```python
from build123d import *

# Parameters (mm, degrees)
SZKIC1_W                    = 28
SZKIC1_H                    = 16
DODANIE_WYCI_GNI_CIE1_DEPTH = 10.4
SZKIC2_R                    = 1.5
WYTNIJ_WYCI_GNI_CIE1_DEPTH  = 10.4
ZAOKR_GLENIE1_R             = 2.5
DODANIE_WYCI_GNI_CIE2_START = -2.5
DODANIE_WYCI_GNI_CIE2_DEPTH = 5
SZKIC5_R                    = 2.229172114
DODANIE_WYCI_GNI_CIE3_DEPTH = 5


with BuildPart() as part:
    # Szkic1 → Dodanie-wyciągnięcie1 (new body)
    with BuildSketch(Plane.XY):
        with Locations((14, 8)):
            Rectangle(SZKIC1_W, SZKIC1_H)
    extrude(amount=DODANIE_WYCI_GNI_CIE1_DEPTH)

    # Szkic2 → Wytnij-wyciągnięcie1 (cut)
    with BuildSketch(Plane.XY.offset(10.4)):
        with Locations((3, 3)):
            Circle(SZKIC2_R)
        with Locations((25, 13)):
            Circle(SZKIC2_R)
    extrude(amount=-WYTNIJ_WYCI_GNI_CIE1_DEPTH, mode=Mode.SUBTRACT)

    # Zaokrąglenie1
    zaokr_glenie1_edges = [part.edges().sort_by_distance(p)[0] for p in [
        (0, 16, 5.2),
        (28, 16, 5.2),
        (28, 0, 5.2),
        (0, 0, 5.2),
    ]]
    fillet(zaokr_glenie1_edges, radius=ZAOKR_GLENIE1_R)

    # Szkic4 → Dodanie-wyciągnięcie2 (add)
    with BuildSketch(Plane.XY.offset(10.4).offset(DODANIE_WYCI_GNI_CIE2_START)):
        Polygon((17.360184227, 16), (-9.374532536, 25.006750185), (-9.835766296, 23.637671029), (15.248549739, 15.186929991), align=None)
    extrude(amount=-DODANIE_WYCI_GNI_CIE2_DEPTH)

    # Szkic5 → Dodanie-wyciągnięcie3 (add)
    with BuildSketch(Plane.XY.offset(7.9)):
        with Locations((-8.559972621, 24.732330309)):
            Circle(SZKIC5_R)
    extrude(amount=-DODANIE_WYCI_GNI_CIE3_DEPTH)


solid = part.part
```
Verification items for the finished model (mm, model axes). A direction names the side the tool comes from. Round coordinates to 2 decimals unless told otherwise and drop trailing zeros. Write each loop counter-clockwise with the first axis right and the second up, starting at its lowest first coordinate (ties: lowest second). Pieces come first, ordered by that corner, then holes. Notation, with made-up numbers: (-18, -6) -> (39, -6) arc R6 ccw to (39, 3) -> close; hole circle Ø2 at (14, 78). An arc over 180 degrees is marked (long way). Write each question's results on one line, items separated by ' | '. Start each with the question number.
1. Depth check by flat-ended pin: P1, Ø3, axis at x = 8.5, z = 3, coming from the +Y side; P2, Ø3.5, axis at x = 9.5, y = 22.5, coming from the -Z side; P3, Ø3.5, axis at x = 25, y = 13, coming from the +Z side; P4, Ø5, axis at y = 6, z = 5.5, coming from the -X side. Enter the tip coordinate at first touch or a pass-through.
2. Cross-section at A-A (z = 7.25). Enter the section's corners in (x, y), then the cut area to 3 significant figures.
3. Material ranges on probe 1 along Y at (x, z) = (25, 7.5); probe 2 along Y at (x, z) = (3, 5); probe 3 along Y at (x, z) = (10, 7), recorded low to high. Write a range as from..to.
4. Draft check along Y on faces 6 (the flat face through (0, 21, 7.9)), 7 (the cylindrical face through (27.248, 0.713, 5.273)), 8 (the cylindrical face through (27.248, 15.287, 5.273)), 9 (the cylindrical face through (3.69, 1.67, 5.27)). Enter one of: +Y half, -Y half, draft (parallel to the pull), parting line (faces both ways), or undercut.
5. Cross-section at C-C (y = 3). Enter the section's corners in (x, z), then the cut area to 3 significant figures.
6. Cross-section at B-B (x = 25). Enter the section's corners in (y, z), then the cut area to 3 significant figures.
7. Cross-section at D-D (x = 3). Enter the section's corners in (y, z).
8. Set-up check for faces 1 (the flat face through (0, 8, 5)), 2 (the flat face through (0, 21, 2.9)), 3 (the flat face through (14, 8, 0)), 4 (the cylindrical face through (0.713, 15.248, 5.273)), 5 (the cylindrical face through (-10.24, 26.2, 5.44)): record each of +Z, -Z, +X, -X, +Y, -Y from which the full face is reachable in a straight line by a thin tool's end or side.
Solutions:
1) P1: stops at y = 19.49 | P2: passes through | P3: stops at z = 10.4 | P4: stops at x = 0
2) outline: (-7.41, 22.82) -> (12.84, 16) -> (2.5, 16) arc R2.5 ccw to (0, 13.5) -> (0, 2.5) arc R2.5 ccw to (2.5, 0) -> (25.5, 0) arc R2.5 ccw to (28, 2.5) -> (28, 13.5) arc R2.5 ccw to (25.5, 16) -> (17.36, 16) -> (-6.45, 24.02) arc R2.23 ccw (long way) to start; hole circle Ø3 at (3, 3); hole circle Ø3 at (25, 13) | area: 478 mm2
3) probe 1: y = 0..11.5, 14.5..16 | probe 2: y = 0..1.5, 4.5..16, 19.31..20.84 | probe 3: y = 0..16, 16.96..18.48
4) face 6: draft | face 7: -Y half | face 8: +Y half | face 9: undercut
5) outline: (0, 0) -> (1.5, 0) -> (1.5, 10.4) -> (0, 10.4) -> close; (4.5, 0) -> (28, 0) -> (28, 10.4) -> (4.5, 10.4) -> close | area: 260 mm2
6) outline: (0, 0) -> (11.5, 0) -> (11.5, 10.4) -> (0, 10.4) -> close; (14.5, 0) -> (16, 0) -> (16, 10.4) -> (14.5, 10.4) -> close | area: 135 mm2
7) outline: (0, 0) -> (1.5, 0) -> (1.5, 10.4) -> (0, 10.4) -> close; (4.5, 0) -> (16, 0) -> (16, 10.4) -> (4.5, 10.4) -> close; (19.31, 2.9) -> (20.84, 2.9) -> (20.84, 7.9) -> (19.31, 7.9) -> close
8) face 1: +Z, -Z, -X, -Y | face 2: -Z, +X, -X, +Y | face 3: -Z, +X, -X, +Y, -Y | face 4: +Z, -Z, -X | face 5: +Z, -Z
